Can you work these out from the drawing? Everything is in mm from the part's minimum corner. Coordinates: 2 decimals unless noted, no trailing zeros. Loops run counter-clockwise (first coordinate to the right, second up) from the corner with the lowest first, then second, coordinate; pieces in that order, holes last.
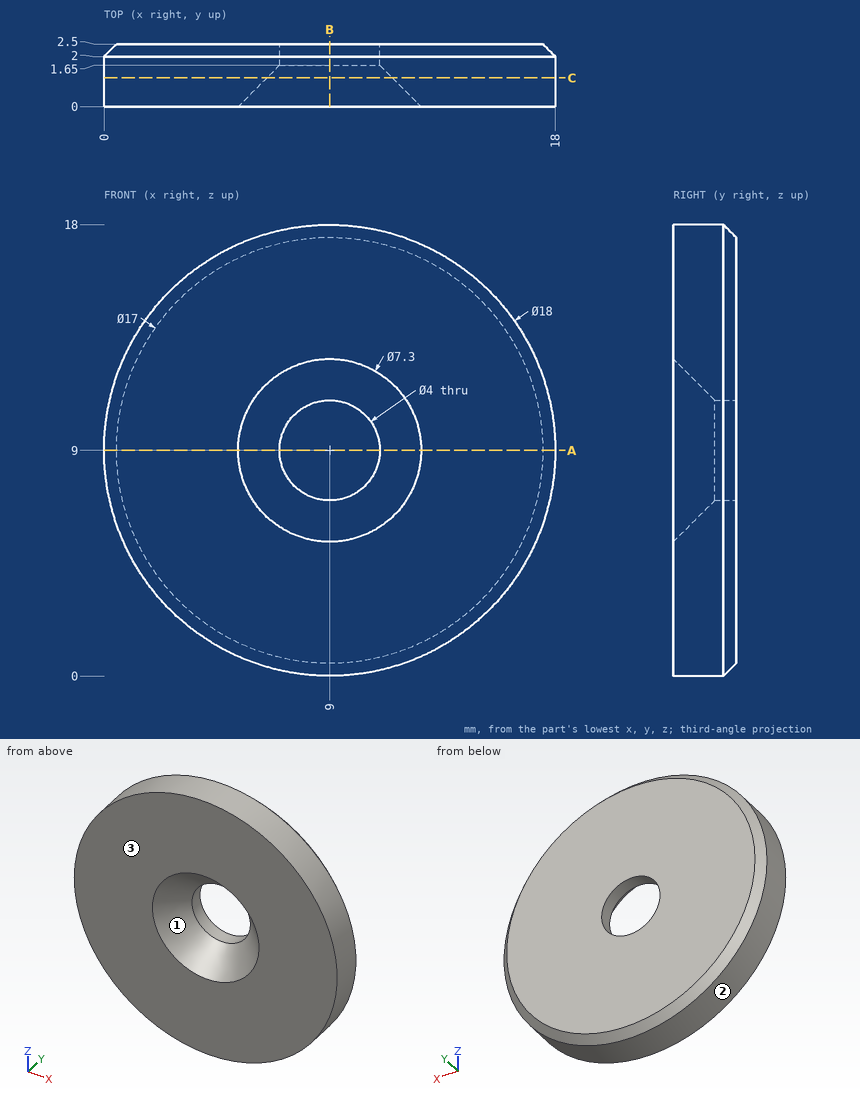
Item 1: Suppose I cut it at C-C, the plane y = 1.15. Please give me the cut outline in (x, z).
Results are:
outline: circle Ø18 at (9, 9); hole circle Ø5 at (9, 9)
Item 2: I'm going to push flat-ended pins straight in: P1, Ø1, axis at y = 1, z = 11, coming from the -X side; P2, Ø1.5, axis at x = 4.5, y = 1, coming from the +Z side; P3, Ø1, axis at y = 0.5, z = 12, coming from the +X side. Where does each tip first touch, or does it pass through?
Results are:
P1: stops at x = 0.13
P2: stops at z = 17.18
P3: stops at x = 17.65
Item 3: Suppose I cut it at A-A, the plane z = 9. Please give me the cut outline in (x, y).
Results are:
outline: (0, 0) - (5.35, 0) - (7, 1.65) - (7, 2.5) - (0.5, 2.5) - (0, 2) - close; (11, 1.65) - (12.65, 0) - (18, 0) - (18, 2) - (17.5, 2.5) - (11, 2.5) - close
Item 4: Suppose I cut it at B-B, the plane x = 9. Please give me the cut outline in (y, z), plus the area to 3 significant figures.
Results are:
outline: (0, 0) - (2, 0) - (2.5, 0.5) - (2.5, 7) - (1.65, 7) - (0, 5.35) - close; (0, 12.65) - (1.65, 11) - (2.5, 11) - (2.5, 17.5) - (2, 18) - (0, 18) - close
area: 32.0 mm2
Item 5: I need wall thicknesses on line 1 along Z through (x, y) = (9, 1.9); line 2 along Z through (x, y) = (8.25, 1.45); line 3 along X through (y, z) = (0.6, 8). Which ranges of each line are inside material? Lowest first, please.
Results are:
line 1: z = 0 to 7, 11 to 18
line 2: z = 0.03 to 6.93, 11.07 to 17.97
line 3: x = 0.06 to 6.12, 11.88 to 17.94
Item 6: We'd pull the mould along Z, two halves only. Please class the marked faces 1, 2 and 3: +Z half, -Z half, draft (parallel to the pull), parting line (faces both ways), or undercut.
Results are:
face 1: undercut
face 2: parting line
face 3: draft
